Drawing for the job (mm, zero at the part's lowest x, y, z). A direction names the side the tool comes from. Round coordinates to 2 decimals unless told otherwise and drop trailing zeros. Loops run counter-clockwise (first coordinate to the right, second up) from the corner with the lowest first, then second, coordinate; pieces in that order, holes last. Notation, with made-up numbers: M 87.25,76.25 L 105.25,76.25 A23 ccw 105.25,97.25 Z; hole C 24,77.5 d1. An arc over 180 degrees is marked long. Put each result on its own line as item: value. Start each with the question number.
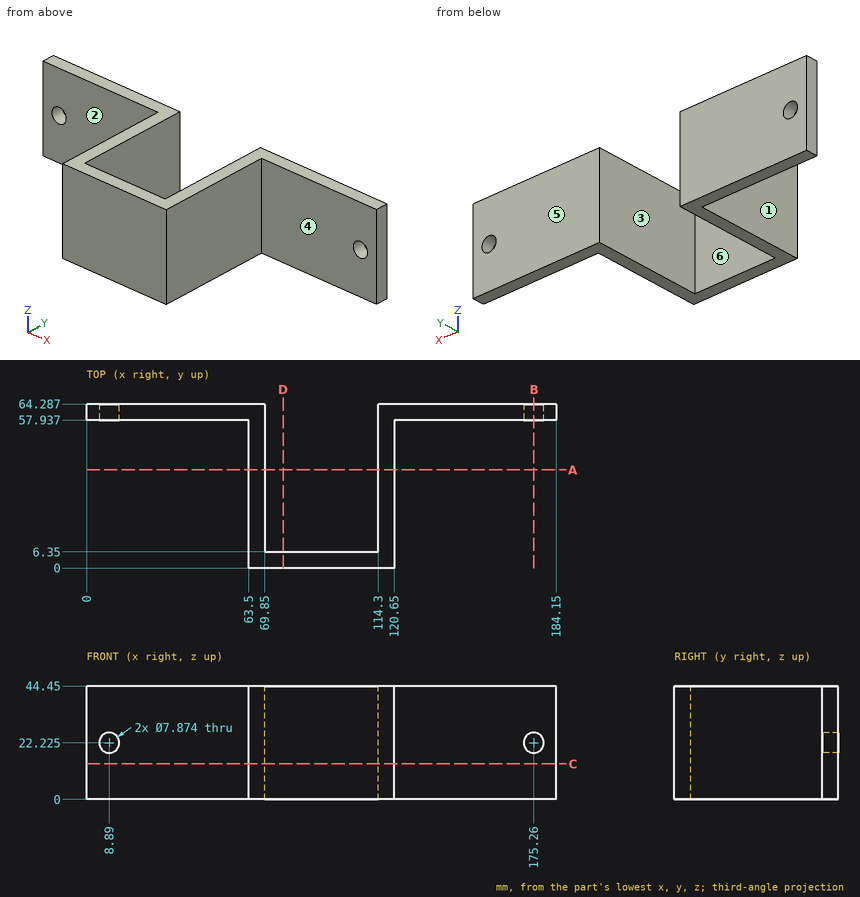
1. Which spindle directions (+Z, -Z, +X, -X, +Y, -Y) get a long thin tool onto all of the face, cutting with end or side? Do the marked faces 4, 5 and 6. Say none if no direction does.
2. Wall check: L1, parallel to Z at x = 175.26, y = 60.25; L2, parallel to X at y = 56, z = 22; L3, parallel to X at y = 58.5, z = 31. Give the ranges that are in metal, low to high.
3. Cut at D-D, the plane x = 77. Give the cut face in (y, z), and give its area (3 significant figures).
4. Cut at A-A, the plane y = 38.5. Give the cut face in (x, z).
5. Cut at C-C, the plane z = 14. Give the cut face in (x, y).
6. Drop flat-ended pins along their axis: pin 1 (1 mm diameter, centred on x = 34.5, z = 12.5, fed in from -Y); pin 2 (13.5 mm diameter, centred on y = 28.5, z = 30.5, fed in from +X); pin 3 (13.5 mm diameter, centred on x = 87, z = 11, fed in from +Y). Give the stop position or say it passes through.
7. Cut at B-B, the plane x = 175.26. Give the cut face in (y, z).
8. Mould opens along X. For the marked faces 1, 2 and 3 say: released by +X, released by -X, zero draft, split by the parting line, or undercut.
Results list:
1. face 4: +Z, -Z, +X, -Y
1. face 5: +Z, -Z, +X, -X, +Y
1. face 6: +Z, -Z, +Y
2. L1: z = 0 to 18.29, 26.16 to 44.45
2. L2: x = 63.5 to 69.85, 114.3 to 120.65
2. L3: x = 0 to 69.85, 114.3 to 184.15
3. outline: M 0,0 L 6.35,0 L 6.35,44.45 L 0,44.45 Z
3. area: 282 mm^2
4. outline: M 63.5,0 L 69.85,0 L 69.85,44.45 L 63.5,44.45 Z; M 114.3,0 L 120.65,0 L 120.65,44.45 L 114.3,44.45 Z
5. outline: M 0,57.94 L 63.5,57.94 L 63.5,0 L 120.65,0 L 120.65,57.94 L 184.15,57.94 L 184.15,64.29 L 114.3,64.29 L 114.3,6.35 L 69.85,6.35 L 69.85,64.29 L 0,64.29 Z
6. pin 1: stops at y = 57.94
6. pin 2: stops at x = 120.65
6. pin 3: stops at y = 6.35
7. outline: M 57.94,0 L 64.29,0 L 64.29,18.29 L 57.94,18.29 Z; M 57.94,26.16 L 64.29,26.16 L 64.29,44.45 L 57.94,44.45 Z
8. face 1: released by -X
8. face 2: zero draft
8. face 3: undercut
